from build123d import *

# Parameters (mm, degrees)
CROQUIS1_W                                   = 208.5
CROQUIS1_H                                   = 80
BRIDA_BASE1_DEPTH                            = 6.35
REDONDEO1_R                                  = 2
TALADRO_DE_MARGEN_PARA_1_41_D                = 6.7564
REFRENTADO_PARA_TORNILLO_TAP_N_CON_C_2_COUNT = 2
REFRENTADO_PARA_TORNILLO_TAP_N_CON_C_2_PITCH = 44
REFRENTADO_PARA_TORNILLO_TAP_N_CON_C_3_COUNT = 2
REFRENTADO_PARA_TORNILLO_TAP_N_CON_C_3_PITCH = 60.827625303
REFRENTADO_PARA_TORNILLO_TAP_N_CON_C_4_COUNT = 2
REFRENTADO_PARA_TORNILLO_TAP_N_CON_C_4_PITCH = 42


# Sheet-metal steps are written as plain solids
with BuildPart() as part:
    # Croquis1 → Brida base1 (new body)
    with BuildSketch(Plane(origin=(0, 0, 0), x_dir=(1, 0, 0), z_dir=(0, 1, 0))):
        with Locations((-45.527777778, -5.555555556)):
            Rectangle(CROQUIS1_W, CROQUIS1_H)
    extrude(amount=-BRIDA_BASE1_DEPTH)

    # Redondeo1
    redondeo1_edges = [part.edges().sort_by_distance(p)[0] for p in [
        (-149.777777778, -3.175, -34.444444444),
        (58.722222222, -3.175, -34.444444444),
        (58.722222222, -3.175, 45.555555556),
        (-149.777777778, -3.175, 45.555555556),
    ]]
    fillet(redondeo1_edges, radius=REDONDEO1_R)

    # Taladro de margen para 1/41 (through all)
    with Locations(Plane(origin=(0, 0, 0), x_dir=(1, 0, 0), z_dir=(0, 1, 0))):
        with Locations((-139.777777778, -25.555555556), (-59.777777778, -25.555555556), (-139.777777778, 14.444444444), (-59.777777778, 14.444444444)):
            Hole(TALADRO_DE_MARGEN_PARA_1_41_D / 2)

    # Croquis9 → Refrentado para tornillo tapón con cabeza plana de clavija de M61 (revolve, cut)
    with BuildSketch(Plane(origin=(-121.777777778, 0, -15.444444444), x_dir=(0, 0, 1), z_dir=(1, 0, 0))):
        Polygon((0, 0), (0, 6.35), (3.3, 6.35), (3.3, 3.42), (6.72, 0), align=None)
    refrentado_para_tornillo_tap_n_con_cabez = revolve(axis=Axis((-121.777777778, 6.35, -15.444444444), (0, -1, 0)), mode=Mode.SUBTRACT)

    # Refrentado para tornillo tap_n con c 2: Refrentado para tornillo tapón con cabeza plana de clavija de M61 ×2
    with Locations(*[(i * REFRENTADO_PARA_TORNILLO_TAP_N_CON_C_2_PITCH, 0, 0) for i in range(1, REFRENTADO_PARA_TORNILLO_TAP_N_CON_C_2_COUNT)]):
        add(refrentado_para_tornillo_tap_n_con_cabez, mode=Mode.SUBTRACT)

    # Refrentado para tornillo tap_n con c 3: Refrentado para tornillo tapón con cabeza plana de clavija de M61 ×2
    with Locations(*[Vector(0.723355544143572, 0, 0.6904757466825007) * (i * REFRENTADO_PARA_TORNILLO_TAP_N_CON_C_3_PITCH) for i in range(1, REFRENTADO_PARA_TORNILLO_TAP_N_CON_C_3_COUNT)]):
        add(refrentado_para_tornillo_tap_n_con_cabez, mode=Mode.SUBTRACT)

    # Refrentado para tornillo tap_n con c 4: Refrentado para tornillo tapón con cabeza plana de clavija de M61 ×2
    with Locations(*[(0, 0, i * REFRENTADO_PARA_TORNILLO_TAP_N_CON_C_4_PITCH) for i in range(1, REFRENTADO_PARA_TORNILLO_TAP_N_CON_C_4_COUNT)]):
        add(refrentado_para_tornillo_tap_n_con_cabez, mode=Mode.SUBTRACT)


solid = part.part
Here's how the part is built. I have some questions about the finished solid (model axes, mm). Coordinates: 2 decimals unless noted, no trailing zeros. Answer in a Markdown table with one row per item.
(1) I want a section at A-A on y = -1. Count the separate pieces of the cut face and the enclosed holes in it, then the cut area to 3 significant figures.
Answer key:
| item | result |
|---|---|
| separate pieces | 1 |
| enclosed holes | 8 |
| area | 16,100 mm^2 |
(2) Thinking about a two-plate mould opening in X: for faces 1 (the face through (-149.778, -3, 6)), 2 (the face through (-57.29, -3.22, 23.27)), 3 (the face through (-47, -3, -34.444)), which applies, +X half, -X half, draft (parallel to the pull), parting line (faces both ways), or undercut?
Answer key:
| item | result |
|---|---|
| face 1 | -X half |
| face 2 | undercut |
| face 3 | draft |
(3) Please list where these lines run through material, in increasing order: probe 1 along X at (y, z) = (-2.75, 28); probe 2 along Z at (x, y) = (-75.5, -2); probe 3 along Y at (x, z) = (-126, -13).
Answer key:
| item | result |
|---|---|
| probe 1 | -149.78 to -142.11, -137.45 to -125.48, -118.08 to -81.48, -74.08 to -62.11, -57.45 to 58.72 |
| probe 2 | -34.44 to -19.58, -11.31 to 22.42, 30.69 to 45.56 |
| probe 3 | -6.35 to -1.84 |
(4) Will these pins go through, and if not, where does the flat tip stop? pin 1 Ø5.5 at (x, z) = (-77.78, -15.44) entering from -Y; pin 2 Ø7.5 at (x, z) = (-121.78, 26.56) entering from +Y; pin 3 Ø10.5 at (x, z) = (-121.78, -15.44) entering from +Y; pin 4 Ø8.5 at (x, z) = (-77.78, 26.56) entering from +Y.
Answer key:
| item | result |
|---|---|
| pin 1 | through |
| pin 2 | y = -2.97 |
| pin 3 | y = -1.47 |
| pin 4 | y = -2.47 |
